```python
from build123d import *

# Parameters (mm, degrees)
SKETCH1_W           = 609.6
SKETCH1_H           = 914.4
BOSS_EXTRUDE1_DEPTH = 4.7625
SKETCH4_W           = 38.1
SKETCH4_H           = 38.1
SKETCH4_W_2         = 25.4
SKETCH4_H_2         = 25.4
BOSS_EXTRUDE2_DEPTH = 25.4


with BuildPart() as part:
    # Sketch1 → Boss-Extrude1 (new body)
    with BuildSketch(Plane(origin=(0, 0, 0), x_dir=(1, 0, 0), z_dir=(0, 1, 0))):
        with Locations((304.8, 457.2)):
            Rectangle(SKETCH1_W, SKETCH1_H)
    extrude(amount=BOSS_EXTRUDE1_DEPTH)

    # Sketch4 → Boss-Extrude2 (add)
    with BuildSketch(Plane(origin=(0, 4.7625, 0), x_dir=(1, 0, 0), z_dir=(0, 1, 0))):
        with Locations((114.3, 711.2)):
            Rectangle(SKETCH4_W, SKETCH4_H)
        with Locations((114.3, 711.2)):
            Rectangle(SKETCH4_W_2, SKETCH4_H_2, mode=Mode.SUBTRACT)
        with Locations((495.3, 711.2)):
            Rectangle(SKETCH4_W, SKETCH4_H)
        with Locations((495.3, 711.2)):
            Rectangle(SKETCH4_W_2, SKETCH4_H_2, mode=Mode.SUBTRACT)
        with Locations((495.3, 203.2)):
            Rectangle(SKETCH4_W, SKETCH4_H)
        with Locations((495.3, 203.2)):
            Rectangle(SKETCH4_W_2, SKETCH4_H_2, mode=Mode.SUBTRACT)
        with Locations((114.3, 203.2)):
            Rectangle(SKETCH4_W, SKETCH4_H)
        with Locations((114.3, 203.2)):
            Rectangle(SKETCH4_W_2, SKETCH4_H_2, mode=Mode.SUBTRACT)
    extrude(amount=BOSS_EXTRUDE2_DEPTH)


solid = part.part
```
The listing builds one solid part. Answer for the finished solid, in the listing's coordinates (mm). A direction names the side the tool comes from. Coordinates: 2 decimals unless noted, no trailing zeros. Write each loop counter-clockwise with the first axis right and the second up, starting at its lowest first coordinate (ties: lowest second). Pieces come first, ordered by that corner, then holes. Notation, with made-up numbers: (42, 36.5) - (65, 36.5) arc R24 cw to (65, 65.5) - close; hole circle Ø5 at (77, 66). An arc over 180 degrees is marked (long way). One line per item, written item: value.
1) For a pull along Z with two mould halves and no side action, classify faces 5 (the flat face through (495, 30.162, -724.2)), 6 (the flat face through (482.6, 17, -203)), 7 (the flat face through (495, 17, -730.25)), 8 (the flat face through (114, 17, -184.15)) as pulls with the +Z half, pulls with the -Z half, needs draft (parallel to the pull), parting line crosses it, or undercut.
Geometry check:
face 5: needs draft
face 6: undercut
face 7: pulls with the -Z half
face 8: pulls with the +Z half
2) Find section A-A (y = 20). Count the separate pieces of the cut face and the enclosed holes in it, and give its area (3 significant figures).
Geometry check:
separate pieces: 4
enclosed holes: 4
area: 3,230 mm2
3) Each of these flat-tipped pins is pushed along its axis until it touches: pin 1 Ø8 at (x, y) = (396, 6.5) entering from -Z; pin 2 Ø12.5 at (x, y) = (109.5, 14) entering from +Z; pin 3 Ø6 at (x, y) = (275.5, 9) entering from -Z; pin 4 Ø3 at (x, z) = (191, -122.5) entering from +Y. Where does it stop, or does it pass through?
Geometry check:
pin 1: stops at z = -914.4
pin 2: stops at z = -184.15
pin 3: passes through
pin 4: stops at y = 4.76
4) Consider line 1 along X through (y, z) = (19, -195); line 2 along Z through (x, y) = (108.5, 24.5); line 3 along Y through (x, z) = (572.5, -495.5). Determine where each line is inside the solid, lowest interval first. Write a range as from..to.
Geometry check:
line 1: x = 95.25..101.6, 127..133.35, 476.25..482.6, 508..514.35
line 2: z = -730.25..-723.9, -698.5..-692.15, -222.25..-215.9, -190.5..-184.15
line 3: y = 0..4.76
5) Find section C-C (x = 244.5). Give the vertices of the cut face in (y, z), and give its area (3 significant figures).
Geometry check:
outline: (0, -914.4) - (4.76, -914.4) - (4.76, 0) - (0, 0) - close
area: 4,350 mm2
6) A tool of negligible diameter and unlimited length cuts with its end or side. For faces 1 (the flat face through (476.25, 17, -203)), 2 (the flat face through (95.25, 17, -711)), 3 (the flat face through (114, 17, -215.9)), 4 (the flat face through (514.35, 17, -203)), from which of +Z, -Z, +X, -X, +Y, -Y can it reach the whole face along a straight path? Write none if from no direction.
Geometry check:
face 1: +Z, -Z, +Y
face 2: +Z, -Z, -X, +Y
face 3: +Y
face 4: +Z, -Z, +X, +Y
7) Find section B-B (z = -400.5). Give the vertices of the cut face in (x, y), and give its area (3 significant figures).
Geometry check:
outline: (0, 0) - (609.6, 0) - (609.6, 4.76) - (0, 4.76) - close
area: 2,900 mm2
